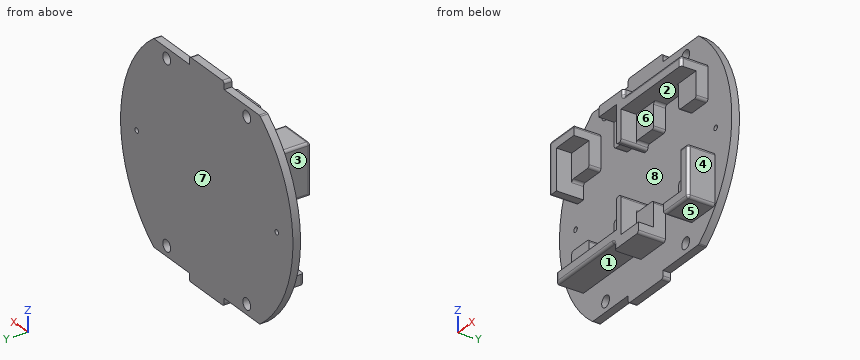
from build123d import *

# Parameters (mm, degrees)
A_BASE_T42_OUTLINE_R       = 2.2479
A_BASE_T42_OUTLINE_R_2     = 1
A_BASE_T42_DEPTH           = 3
OUTER_RIM_CUT_DEPTH        = 68.299702823
SKETCH2_W                  = 20
SKETCH2_H                  = 3
FLANGES_DEPTH              = 3
CONTOURING_R               = 1
SKETCH3_W                  = 15
SKETCH3_H                  = 3
BASE_SUPPORTS_DEPTH        = 3
BASE_SUPPORTS_CHAMFER_SIZE = 3
SKETCH10_W                 = 15
SKETCH10_H                 = 6
CUT_EXTRUDE1_DEPTH         = 10
SKETCH9_W                  = 10
SKETCH9_H                  = 10
BOSS_EXTRUDE1_DEPTH        = 4.6
BOSS_EXTRUDE2_DEPTH        = 10.6
FILLET1_R                  = 1


# Read off the part's stored shape, not the designer's step: a_base_t42
with BuildPart() as part:
    # a_base_t42 outline → a_base_t42 (new body)
    with BuildSketch(Plane(origin=(0, 0, 0), x_dir=(1, 0, 0), z_dir=(0, 1, 0))):
        with BuildLine():
            ThreePointArc((31.5, -42), (52.5, 0), (31.5, 42))
            Line((31.5, 42), (-31.5, 42))
            ThreePointArc((-31.5, 42), (-52.5, 0), (-31.5, -42))
            Line((-31.5, -42), (31.5, -42))
        make_face()
        with Locations((-23, -35)):
            Circle(A_BASE_T42_OUTLINE_R, mode=Mode.SUBTRACT)
        with Locations((23, -35)):
            Circle(A_BASE_T42_OUTLINE_R, mode=Mode.SUBTRACT)
        with Locations((-40.25, 0)):
            Circle(A_BASE_T42_OUTLINE_R_2, mode=Mode.SUBTRACT)
        with Locations((-23, 35)):
            Circle(A_BASE_T42_OUTLINE_R, mode=Mode.SUBTRACT)
        with Locations((40.25, 0)):
            Circle(A_BASE_T42_OUTLINE_R_2, mode=Mode.SUBTRACT)
        with Locations((23, 35)):
            Circle(A_BASE_T42_OUTLINE_R, mode=Mode.SUBTRACT)
    extrude(amount=A_BASE_T42_DEPTH)

    # Sketch1 → Outer Rim Cut (cut, through all)
    with BuildSketch(Plane.XZ):
        with BuildLine():
            Line((31.5, 42), (-31.5, 42))
            ThreePointArc((-31.5, 42), (-52.5, 0), (-31.5, -42))
            Line((-31.5, -42), (31.5, -42))
            ThreePointArc((31.5, -42), (52.5, 0), (31.5, 42))
        make_face()
        with BuildLine():
            Line((30.483602149, 39), (-30.483602149, 39))
            ThreePointArc((-30.483602149, 39), (-49.5, 0), (-30.483602149, -39))
            Line((-30.483602149, -39), (30.483602149, -39))
            ThreePointArc((30.483602149, -39), (49.5, 0), (30.483602149, 39))
        make_face(mode=Mode.SUBTRACT)
    extrude(amount=-OUTER_RIM_CUT_DEPTH, mode=Mode.SUBTRACT)

    # Sketch2 → Flanges (add)
    with BuildSketch(Plane.XZ):
        with Locations((0, -40.5)):
            Rectangle(SKETCH2_W, SKETCH2_H)
        with Locations((0, 40.5)):
            Rectangle(SKETCH2_W, SKETCH2_H)
    extrude(amount=-FLANGES_DEPTH)

    # Contouring
    contouring_edges = [part.edges().sort_by_distance(p)[0] for p in [
        (30.483602149, 1.5, -39),
        (-30.483602149, 1.5, -39),
        (10, 1.5, -42),
        (-10, 1.5, -42),
        (30.483602149, 1.5, 39),
        (-30.483602149, 1.5, 39),
        (10, 1.5, 42),
        (-10, 1.5, 42),
    ]]
    fillet(contouring_edges, radius=CONTOURING_R)

    # Sketch3 → Base Supports (add)
    with BuildSketch(Plane.XZ):
        with Locations((0, -27)):
            Rectangle(SKETCH3_W, SKETCH3_H)
        with Locations((0, 27)):
            Rectangle(SKETCH3_W, SKETCH3_H)
    extrude(amount=BASE_SUPPORTS_DEPTH)

    # Base Supports Chamfer
    base_supports_chamfer_edges = [part.edges().sort_by_distance(p)[0] for p in [
        (0, 0, 28.5),
        (0, 0, -28.5),
    ]]
    chamfer(base_supports_chamfer_edges, length=BASE_SUPPORTS_CHAMFER_SIZE - 0.0001)  # a hair under: the kernel refuses the full size

    # Sketch10 → Cut-Extrude1 (cut)
    with BuildSketch(Plane.XZ):
        with Locations((0, 28.5)):
            Rectangle(SKETCH10_W, SKETCH10_H)
        with Locations((0, -28.5)):
            Rectangle(SKETCH10_W, SKETCH10_H)
    extrude(amount=CUT_EXTRUDE1_DEPTH, mode=Mode.SUBTRACT)

    # Sketch9 → Boss-Extrude1 (add)
    with BuildSketch(Plane.XZ):
        with Locations((6.35, 16.95)):
            Rectangle(SKETCH9_W, SKETCH9_H)
        with Locations((30.75, 16.95)):
            Rectangle(SKETCH9_W, SKETCH9_H)
        with Locations((30.75, -19.95)):
            Rectangle(SKETCH9_W, SKETCH9_H)
        with Locations((6.35, -19.95)):
            Rectangle(SKETCH9_W, SKETCH9_H)
        with Locations((-6.35, -16.95)):
            Rectangle(SKETCH9_W, SKETCH9_H)
        with Locations((-6.35, 19.95)):
            Rectangle(SKETCH9_W, SKETCH9_H)
        with Locations((-30.75, 19.95)):
            Rectangle(SKETCH9_W, SKETCH9_H)
        with Locations((-30.75, -16.95)):
            Rectangle(SKETCH9_W, SKETCH9_H)
    extrude(amount=BOSS_EXTRUDE1_DEPTH)

    # Sketch11 → Boss-Extrude2 (add)
    with BuildSketch(Plane.XZ):
        Polygon((35.75, -24.95), (35.75, -8.95), (39.75, -8.95), (39.75, -28.95), (25.75, -28.95), (25.75, -24.95), align=None)
        Polygon((-2.65, -28.95), (-2.65, -25.95), (-35.75, -25.95), (-35.75, -21.95), (-1.35, -21.95), (-1.35, -9.95), (1.35, -9.95), (1.35, -24.95), (11.35, -24.95), (11.35, -28.95), align=None)
        Polygon((-1.35, 24.95), (-11.35, 24.95), (-11.35, 28.95), (2.65, 28.95), (2.65, 25.95), (35.75, 25.95), (35.75, 21.95), (1.35, 21.95), (1.35, 9.95), (-1.35, 9.95), align=None)
        Polygon((-35.75, 24.95), (-35.75, 8.95), (-39.75, 8.95), (-39.75, 28.95), (-25.75, 28.95), (-25.75, 24.95), align=None)
    extrude(amount=BOSS_EXTRUDE2_DEPTH)

    # Fillet1
    fillet1_edges = [part.edges().sort_by_distance(p)[0] for p in [
        (2.65, -10.6, 27.45),
        (-2.65, -10.6, -27.45),
        (2.65, -5.3, 25.95),
        (-39.75, -5.3, 28.95),
        (-39.75, -5.3, 8.95),
        (-1.35, -2.3, 14.95),
        (-11.35, -2.3, 14.95),
        (-25.75, -2.3, 14.95),
        (-35.75, -2.3, 14.95),
        (-1.35, -2.3, -11.95),
        (-11.35, -2.3, -21.95),
        (-11.35, -2.3, -11.95),
        (-25.75, -2.3, -21.95),
        (35.75, -2.3, 11.95),
        (-35.75, -2.3, -11.95),
        (-25.75, -2.3, -11.95),
        (-35.75, -10.6, -23.95),
        (39.75, -10.6, -18.95),
        (37.75, -10.6, -8.95),
        (35.75, -10.6, 23.95),
        (19.2, -10.6, 25.95),
        (35.75, -5.3, 25.95),
        (25.75, -2.3, 11.95),
        (25.75, -2.3, 21.95),
        (11.35, -2.3, 21.95),
        (1.35, -2.3, 11.95),
        (11.35, -2.3, 11.95),
        (-1.35, -5.3, 9.95),
        (1.35, -5.3, 9.95),
        (1.35, -5.3, -9.95),
        (-1.35, -5.3, -9.95),
        (1.35, -2.3, -14.95),
        (11.35, -2.3, -14.95),
        (25.75, -2.3, -14.95),
        (35.75, -2.3, -14.95),
        (39.75, -5.3, -8.95),
        (39.75, -5.3, -28.95),
        (32.75, -10.6, -28.95),
        (-2.65, -5.3, -25.95),
        (-19.2, -10.6, -25.95),
        (-39.75, -10.6, 18.95),
        (-32.75, -10.6, 28.95),
        (-11.35, -5.3, 28.95),
        (-25.75, -5.3, 28.95),
        (11.35, -5.3, -28.95),
        (25.75, -5.3, -28.95),
    ]]
    fillet(fillet1_edges, radius=FILLET1_R - 0.0001)  # a hair under: the kernel refuses the full size


solid = part.part
Geometry: final body of the model. Coordinates: model frame, mm. Face numbers are marked on the shaded views. A direction names the side the tool comes from. Round coordinates to 2 decimals unless told otherwise and drop trailing zeros. Order: outer loops, then holes, each group sorted by start corner. A loop starts at its lowest first (then second) coordinate and runs counter-clockwise, first axis right, second up. Notation, with made-up numbers: (78.25, 64.5) - (109.25, 64.5) arc R27 ccw to (109.25, 88.5) - close; hole circle Ø11 at (-6, 10). An arc over 180 degrees is marked (long way). Write each question's results on one line, items separated by ' | '.
Item 1: Section D-D, the plane z = -23.5. Return the cut outline in (x, y), and give its area (3 significant figures).
Completed:
outline: (-43.57, 0) - (-35.75, 0) - (-35.75, -9.6) arc R1 ccw to (-34.75, -10.6) - (1.35, -10.6) - (1.35, -4.6) - (11.35, -4.6) - (11.35, 0) - (25.75, 0) - (25.75, -4.6) - (35.75, -4.6) - (35.75, -10.6) - (38.75, -10.6) arc R1 ccw to (39.75, -9.6) - (39.75, 0) - (43.57, 0) - (43.57, 3) - (-43.57, 3) - close | area: 789 mm^2
Item 2: Reachability of the marked faces 4, 5, 6, 7 and 8 from +Z, -Z, +X, -X, +Y, -Y: full face, straight path, thin tool, end or side. Return the list, or none.
Completed:
face 4: +Z, -Z, +X, -Y | face 5: -Z, +X, -X, -Y | face 6: +X, -Y | face 7: +Z, -Z, +X, -X, +Y | face 8: -Y
Item 3: Mould query, pull axis Z, two halves, no side actions, for the marked faces 1, 2 and 3. Classes: pulls with the +Z half, pulls with the -Z half, needs draft (parallel to the pull), parting line crosses it, or undercut.
Completed:
face 1: pulls with the -Z half | face 2: undercut | face 3: needs draft
Item 4: Material intervals for line 1 along X through (y, z) = (1.85, 0); line 2 along Z through (x, y) = (-23, 1.8); line 3 along Z through (x, y) = (29.5, -7.25), sorted ascending. Write a range as [from, to].
Completed:
line 1: [-49.5, -41.25], [-39.25, 39.25], [41.25, 49.5] | line 2: [-39, -37.25], [-32.75, 32.75], [37.25, 39] | line 3: [-28.95, -24.95], [21.95, 25.95]
Item 5: Section C-C, the plane y = -6. State how many separate pieces and enclosed holes the cut face has, and give its area (3 significant figures).
Completed:
separate pieces: 4 | enclosed holes: 0 | area: 703 mm^2
Item 6: First-contact query: pin 1 Ø0.6 at (x, y) = (0, -4.5) entering from +Z; pin 2 Ø5.5 at (y, z) = (-4.5, 15) entering from +X; pin 3 Ø2 at (x, z) = (31, 19) entering from -Y; pin 4 Ø1.6 at (x, z) = (-40.25, 0) entering from +Y. Flat tips, straight axial feed; report the tip coordinate or a pass-through.
Completed:
pin 1: z = 28.95 | pin 2: x = 35.75 | pin 3: y = -4.6 | pin 4: through
Item 7: Section B-B, the plane z = -35. Return the cut outline in (x, y).
Completed:
outline: (-35, 0) - (-25.25, 0) - (-25.25, 3) - (-35, 3) - close; (-20.75, 0) - (20.75, 0) - (20.75, 3) - (-20.75, 3) - close; (25.25, 0) - (35, 0) - (35, 3) - (25.25, 3) - close
Item 8: Section A-A, the plane x = 23. Return the cut outline in (y, z).
Completed:
outline: (-10.6, 21.95) - (0, 21.95) - (0, -32.75) - (3, -32.75) - (3, 32.75) - (0, 32.75) - (0, 25.95) - (-9.6, 25.95) arc R1 ccw to (-10.6, 24.95) - close; (0, -39) - (3, -39) - (3, -37.25) - (0, -37.25) - close; (0, 37.25) - (3, 37.25) - (3, 39) - (0, 39) - close
